from build123d import *

# Parameters (mm, degrees)
ESQUISSE1_W        = 86
ESQUISSE1_H        = 70
ESQUISSE1_R        = 2
BOSS_EXTRU_1_DEPTH = 10


with BuildPart() as part:
    # Esquisse1 → Boss.-Extru.1 (new body)
    with BuildSketch(Plane.XY):
        with Locations((43, -35)):
            Rectangle(ESQUISSE1_W, ESQUISSE1_H)
        with Locations((3, -17.5)):
            Circle(ESQUISSE1_R, mode=Mode.SUBTRACT)
        with Locations((3, -52.5)):
            Circle(ESQUISSE1_R, mode=Mode.SUBTRACT)
        with Locations((36.4, -52.5)):
            Circle(ESQUISSE1_R, mode=Mode.SUBTRACT)
        with Locations((36.4, -17.5)):
            Circle(ESQUISSE1_R, mode=Mode.SUBTRACT)
        with Locations(Location((49.6, -52.5, 0), (0, 0, 180))):
            Circle(ESQUISSE1_R, mode=Mode.SUBTRACT)
        with Locations(Location((83, -52.5, 0), (0, 0, 180))):
            Circle(ESQUISSE1_R, mode=Mode.SUBTRACT)
        with Locations(Location((83, -17.5, 0), (0, 0, 180))):
            Circle(ESQUISSE1_R, mode=Mode.SUBTRACT)
        with Locations(Location((49.6, -17.5, 0), (0, 0, 180))):
            Circle(ESQUISSE1_R, mode=Mode.SUBTRACT)
    extrude(amount=BOSS_EXTRU_1_DEPTH)


solid = part.part
The model under review builds one solid part; all positions refer to its coordinate system, in mm. Coordinates: 2 decimals unless noted, no trailing zeros. Loops run counter-clockwise (first coordinate to the right, second up) from the corner with the lowest first, then second, coordinate; pieces in that order, holes last. Notation, with made-up numbers: (79, 88.5) -> (124, 88.5) arc R27 ccw to (124, 117.5) -> close; hole circle Ø1 at (24, -14.75). An arc over 180 degrees is marked (long way). Use a Markdown table: item, result. Add a question column.
1. To check wall thickness, follow line 1 (Y direction, x = 36.4, z = 7.75); line 2 (X direction, y = -19, z = 9.25); line 3 (Y direction, x = 82, z = 1.5). State the ranges of each line that lie inside material, in increasing order.
2. Add section A-A on x = 49.6. Write out the cut boundary in (y, z).
3. Add section C-C on z = 3. Give the number of separate pieces and of enclosed holes in the cut face, plus the area to 3 significant figures.
4. Clearance check with flat-ended pins moving along their axes: pin 1 Ø6.5 at (x, y) = (83, -52.5) entering from +Z; pin 2 Ø2.5 at (x, y) = (3, -52.5) entering from -Z. State where each tip first meets the part, or that it passes through.
5. Draft analysis for pull direction X (two halves, no side actions). For faces 1 (the face through (86, -35, 5)), 2 (the face through (0, -35, 5)), 3 (the face through (49.86, -19.483, 4.93)), state which applies: pulls with the +X half, pulls with the -X half, needs draft (parallel to the pull), parting line crosses it, or undercut.
6. Add section B-B on y = -52.5. Write out the cut boundary in (x, z), plus the area to 3 significant figures.
Returned:
| question | item | result |
|---|---|---|
| 1 | line 1 | y = -70 to -54.5, -50.5 to -19.5, -15.5 to 0 |
| 1 | line 2 | x = 0 to 1.68, 4.32 to 35.08, 37.72 to 48.28, 50.92 to 81.68, 84.32 to 86 |
| 1 | line 3 | y = -70 to -54.23, -50.77 to -19.23, -15.77 to 0 |
| 2 | outline | (-70, 0) -> (-54.5, 0) -> (-54.5, 10) -> (-70, 10) -> close; (-50.5, 0) -> (-19.5, 0) -> (-19.5, 10) -> (-50.5, 10) -> close; (-15.5, 0) -> (0, 0) -> (0, 10) -> (-15.5, 10) -> close |
| 3 | separate pieces | 1 |
| 3 | enclosed holes | 8 |
| 3 | area | 5,920 mm² |
| 4 | pin 1 | stops at z = 10 |
| 4 | pin 2 | passes through |
| 5 | face 1 | pulls with the +X half |
| 5 | face 2 | pulls with the -X half |
| 5 | face 3 | undercut |
| 6 | outline | (0, 0) -> (1, 0) -> (1, 10) -> (0, 10) -> close; (5, 0) -> (34.4, 0) -> (34.4, 10) -> (5, 10) -> close; (38.4, 0) -> (47.6, 0) -> (47.6, 10) -> (38.4, 10) -> close; (51.6, 0) -> (81, 0) -> (81, 10) -> (51.6, 10) -> close; (85, 0) -> (86, 0) -> (86, 10) -> (85, 10) -> close |
| 6 | area | 700 mm² |
